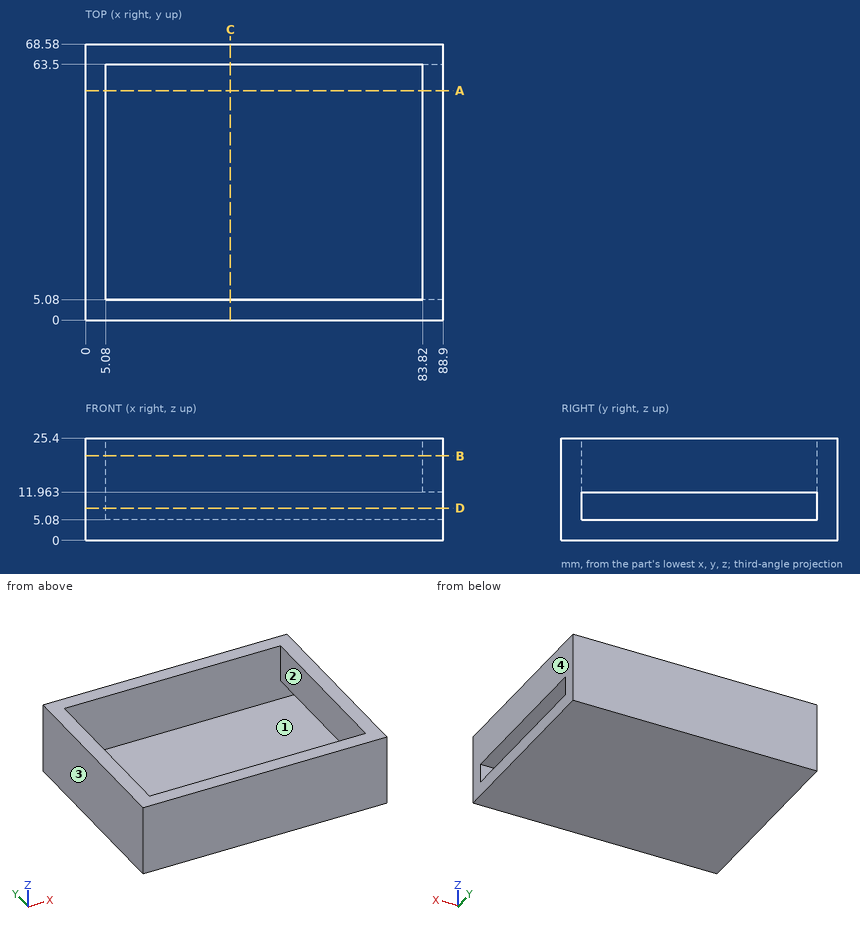
For this review, use the dimensioned drawing (mm, ordinates from the lowest corner) and the shaded views. Round coordinates to 2 decimals unless told otherwise and drop trailing zeros. Order: outer loops, then holes, each group sorted by start corner. A loop starts at its lowest first (then second) coordinate and runs counter-clockwise, first axis right, second up. Notation, with made-up numbers: (-10.75, 52) -> (-0.75, 52) arc R31 cw to (-0.75, 89) -> close; hole circle Ø7 at (54.25, 68.25). An arc over 180 degrees is marked (long way). One line per item, written item: value. Start each with the question number.
Q1. Take a section at D-D (z = 8). Write out the cut boundary in (x, y), and give its area (3 significant figures).
Q2. Wall thickness on line 1 (Y direction, x = 9, z = 10.5); line 2 (X direction, y = 34.5, z = 12.75); line 3 (X direction, y = 52.5, z = 7): over which ranges is each line inside the solid? List them lowest first.
Q3. Take a section at A-A (y = 57). Write out the cut boundary in (x, z), and give its area (3 significant figures).
Q4. Mouldability with a two-part tool opening along X and no side actions: class the marked faces 1, 2, 3 and 4 as released by +X, released by -X, zero draft, split by the parting line, or undercut.
Q5. Take a section at B-B (z = 21). Write out the cut boundary in (x, y).
Q6. Take a section at C-C (x = 36). Write out the cut boundary in (y, z).
Reported:
1. outline: (0, 0) -> (88.9, 0) -> (88.9, 5.08) -> (5.08, 5.08) -> (5.08, 63.5) -> (88.9, 63.5) -> (88.9, 68.58) -> (0, 68.58) -> close
1. area: 1,200 mm2
2. line 1: y = 0 to 5.08, 63.5 to 68.58
2. line 2: x = 0 to 5.08, 83.82 to 88.9
2. line 3: x = 0 to 5.08
3. outline: (0, 0) -> (88.9, 0) -> (88.9, 5.08) -> (5.08, 5.08) -> (5.08, 25.4) -> (0, 25.4) -> close; (83.82, 11.96) -> (88.9, 11.96) -> (88.9, 25.4) -> (83.82, 25.4) -> close
3. area: 623 mm2
4. face 1: zero draft
4. face 2: undercut
4. face 3: released by -X
4. face 4: released by +X
5. outline: (0, 0) -> (88.9, 0) -> (88.9, 68.58) -> (0, 68.58) -> close; hole (5.08, 5.08) -> (83.82, 5.08) -> (83.82, 63.5) -> (5.08, 63.5) -> close
6. outline: (0, 0) -> (68.58, 0) -> (68.58, 25.4) -> (63.5, 25.4) -> (63.5, 5.08) -> (5.08, 5.08) -> (5.08, 25.4) -> (0, 25.4) -> close
